Could you check a few things on this model? Use its own coordinates, in mm. Round coordinates to 2 decimals unless told otherwise and drop trailing zeros. Write each loop counter-clockwise with the first axis right and the second up, starting at its lowest first coordinate (ties: lowest second). Pieces come first, ordered by that corner, then holes. Notation, with made-up numbers: (40, -39.75) -> (88, -39.75) arc R16 cw to (88, -15.75) -> close; hole circle Ø5 at (79, -40). An arc over 180 degrees is marked (long way). Return JSON: item names as keys, results as strings.
from build123d import *

# Parameters (mm, degrees)
SKETCH_1_R      = 2
SKETCH_1_R_2    = 1.5
SKETCH_1_R_3    = 8
EXTRUDE_1_DEPTH = 2


with BuildPart() as part:
    # 草图1 → 凸台-拉伸1 (new body)
    with BuildSketch(Plane(origin=(0, 0, 0), x_dir=(1, 0, 0), z_dir=(0, 1, 0))):
        with BuildLine():
            Line((394.734384308, 186.437991397), (394.734384308, 47.57418904))
            ThreePointArc((394.734384308, 47.57418904), (392.977024848, 43.331548206), (388.734383891, 41.574189041))
            Line((388.734383891, 41.574189041), (280.734383891, 41.574189041))
            ThreePointArc((280.734383891, 41.574189041), (276.491743156, 43.331548327), (274.734383818, 47.57418904))
            Line((274.734383818, 47.57418904), (274.734383818, 186.437990955))
            ThreePointArc((274.734383818, 186.437990955), (274.374769614, 188.48397581), (273.339034443, 190.284705955))
            ThreePointArc((273.339034443, 190.284705955), (336.622100005, 321.857720451), (394.944496295, 188.011903851))
            ThreePointArc((394.944496295, 188.011903851), (394.787144273, 187.231928967), (394.734384308, 186.437991397))
        make_face()
        with Locations(Location((370.121603429, 276.574189041, 0), (0, 0, 270))):
            Circle(SKETCH_1_R, mode=Mode.SUBTRACT)
        with Locations(Location((369.73616956, 206.574189041, 0), (0, 0, 270))):
            Circle(SKETCH_1_R, mode=Mode.SUBTRACT)
        with Locations(Location((300.121603429, 206.574189041, 0), (0, 0, 270))):
            Circle(SKETCH_1_R, mode=Mode.SUBTRACT)
        with Locations(Location((313.734383891, 157.57418904, 0), (0, 0, 270))):
            Circle(SKETCH_1_R_2, mode=Mode.SUBTRACT)
        with Locations(Location((355.734383891, 157.57418904, 0), (0, 0, 270))):
            Circle(SKETCH_1_R_2, mode=Mode.SUBTRACT)
        with Locations(Location((380.234383891, 133.07418904, 0), (0, 0, 270))):
            Circle(SKETCH_1_R_2, mode=Mode.SUBTRACT)
        with Locations(Location((380.234383891, 158.07418904, 0), (0, 0, 270))):
            Circle(SKETCH_1_R_2, mode=Mode.SUBTRACT)
        with Locations(Location((364.734383891, 61.57418904, 0), (0, 0, 270))):
            Circle(SKETCH_1_R_2, mode=Mode.SUBTRACT)
        with Locations(Location((388.734383891, 61.57418904, 0), (0, 0, 270))):
            Circle(SKETCH_1_R_2, mode=Mode.SUBTRACT)
        with Locations(Location((364.734383891, 91.57418904, 0), (0, 0, 270))):
            Circle(SKETCH_1_R_2, mode=Mode.SUBTRACT)
        with Locations(Location((388.734383891, 91.57418904, 0), (0, 0, 270))):
            Circle(SKETCH_1_R_2, mode=Mode.SUBTRACT)
        with Locations(Location((304.734383891, 61.57418904, 0), (0, 0, 270))):
            Circle(SKETCH_1_R_2, mode=Mode.SUBTRACT)
        with Locations(Location((280.734383891, 61.57418904, 0), (0, 0, 270))):
            Circle(SKETCH_1_R_2, mode=Mode.SUBTRACT)
        with Locations(Location((304.734383891, 91.57418904, 0), (0, 0, 270))):
            Circle(SKETCH_1_R_2, mode=Mode.SUBTRACT)
        with Locations(Location((280.734383891, 91.57418904, 0), (0, 0, 270))):
            Circle(SKETCH_1_R_2, mode=Mode.SUBTRACT)
        with Locations(Location((334.734383891, 316.57418904, 0), (0, 0, 270))):
            Circle(SKETCH_1_R_2, mode=Mode.SUBTRACT)
        with Locations(Location((281.701375302, 294.607197629, 0), (0, 0, 270))):
            Circle(SKETCH_1_R_2, mode=Mode.SUBTRACT)
        with Locations(Location((259.734383891, 241.574189041, 0), (0, 0, 270))):
            Circle(SKETCH_1_R_2, mode=Mode.SUBTRACT)
        with Locations(Location((281.701375302, 188.541180451, 0), (0, 0, 270))):
            Circle(SKETCH_1_R_2, mode=Mode.SUBTRACT)
        with Locations(Location((387.76739248, 188.541180451, 0), (0, 0, 270))):
            Circle(SKETCH_1_R_2, mode=Mode.SUBTRACT)
        with Locations(Location((409.734383891, 241.574189041, 0), (0, 0, 270))):
            Circle(SKETCH_1_R_2, mode=Mode.SUBTRACT)
        with Locations(Location((387.76739248, 294.607197629, 0), (0, 0, 270))):
            Circle(SKETCH_1_R_2, mode=Mode.SUBTRACT)
        with Locations(Location((322.734383891, 306.575974709, 0), (0, 0, 270))):
            Circle(SKETCH_1_R_2, mode=Mode.SUBTRACT)
        with Locations(Location((346.734383891, 306.575974709, 0), (0, 0, 270))):
            Circle(SKETCH_1_R_2, mode=Mode.SUBTRACT)
        with Locations(Location((322.734383891, 276.575974709, 0), (0, 0, 270))):
            Circle(SKETCH_1_R_2, mode=Mode.SUBTRACT)
        with Locations(Location((346.734383891, 276.575974709, 0), (0, 0, 270))):
            Circle(SKETCH_1_R_2, mode=Mode.SUBTRACT)
        with Locations(Location((334.734383891, 309.57418904, 0), (0, 0, 270))):
            Circle(SKETCH_1_R_2, mode=Mode.SUBTRACT)
        with Locations(Location((341.734383891, 309.57418904, 0), (0, 0, 270))):
            Circle(SKETCH_1_R_2, mode=Mode.SUBTRACT)
        with Locations(Location((327.734383891, 309.57418904, 0), (0, 0, 270))):
            Circle(SKETCH_1_R_2, mode=Mode.SUBTRACT)
        with Locations(Location((302.217879596, 301.607197629, 0), (0, 0, 270))):
            Circle(SKETCH_1_R_2, mode=Mode.SUBTRACT)
        with Locations(Location((302.217879596, 294.607197629, 0), (0, 0, 270))):
            Circle(SKETCH_1_R_2, mode=Mode.SUBTRACT)
        with Locations(Location((309.217879596, 294.607197629, 0), (0, 0, 270))):
            Circle(SKETCH_1_R_2, mode=Mode.SUBTRACT)
        with Locations(Location((295.217879596, 294.607197629, 0), (0, 0, 270))):
            Circle(SKETCH_1_R_2, mode=Mode.SUBTRACT)
        with Locations(Location((367.250888185, 301.607197629, 0), (0, 0, 270))):
            Circle(SKETCH_1_R_2, mode=Mode.SUBTRACT)
        with Locations(Location((367.250888185, 294.607197629, 0), (0, 0, 270))):
            Circle(SKETCH_1_R_2, mode=Mode.SUBTRACT)
        with Locations(Location((360.250888185, 294.607197629, 0), (0, 0, 270))):
            Circle(SKETCH_1_R_2, mode=Mode.SUBTRACT)
        with Locations(Location((374.250888185, 294.607197629, 0), (0, 0, 270))):
            Circle(SKETCH_1_R_2, mode=Mode.SUBTRACT)
        with Locations(Location((289.234383891, 133.07418904, 0), (0, 0, 270))):
            Circle(SKETCH_1_R_2, mode=Mode.SUBTRACT)
        with Locations(Location((289.234383891, 158.07418904, 0), (0, 0, 270))):
            Circle(SKETCH_1_R_2, mode=Mode.SUBTRACT)
        with Locations(Location((304.734383891, 47.57418904, 0), (0, 0, 270))):
            Circle(SKETCH_1_R_2, mode=Mode.SUBTRACT)
        with Locations(Location((364.734383891, 47.57418904, 0), (0, 0, 270))):
            Circle(SKETCH_1_R_2, mode=Mode.SUBTRACT)
        with Locations(Location((335.121603429, 47.57418904, 0), (0, 0, 270))):
            Circle(SKETCH_1_R_2, mode=Mode.SUBTRACT)
        with Locations(Location((334.734383891, 136.57418904, 0), (0, 0, 270))):
            Circle(SKETCH_1_R_3, mode=Mode.SUBTRACT)
        with Locations(Location((300.121603429, 276.574189041, 0), (0, 0, 270))):
            Circle(SKETCH_1_R, mode=Mode.SUBTRACT)
        with Locations(Location((367.121603429, 157.57418904, 0), (0, 0, 270))):
            Circle(SKETCH_1_R_2, mode=Mode.SUBTRACT)
        with Locations(Location((367.121603429, 99.57418904, 0), (0, 0, 270))):
            Circle(SKETCH_1_R_2, mode=Mode.SUBTRACT)
        with Locations(Location((303.121603429, 157.57418904, 0), (0, 0, 270))):
            Circle(SKETCH_1_R_2, mode=Mode.SUBTRACT)
        with Locations(Location((303.121603429, 99.57418904, 0), (0, 0, 270))):
            Circle(SKETCH_1_R_2, mode=Mode.SUBTRACT)
        with BuildLine():
            Line((354.234383891, 115.57418904), (354.234383891, 89.57418904))
            ThreePointArc((354.234383891, 89.57418904), (355.734383891, 88.07418904), (357.234383891, 89.57418904))
            Line((357.234383891, 89.57418904), (357.234383891, 115.57418904))
            ThreePointArc((357.234383891, 115.57418904), (355.734383891, 117.07418904), (354.234383891, 115.57418904))
        make_face(mode=Mode.SUBTRACT)
        with BuildLine():
            Line((312.234383891, 115.57418904), (312.234383891, 89.57418904))
            ThreePointArc((312.234383891, 89.57418904), (313.734383891, 88.07418904), (315.234383891, 89.57418904))
            Line((315.234383891, 89.57418904), (315.234383891, 115.57418904))
            ThreePointArc((315.234383891, 115.57418904), (313.734383891, 117.07418904), (312.234383891, 115.57418904))
        make_face(mode=Mode.SUBTRACT)
        with BuildLine():
            Line((373.73438389, 46.07418904), (388.734383949, 46.07418904))
            ThreePointArc((388.734383949, 46.07418904), (390.234384308, 47.574188681), (388.734384668, 49.07418904))
            Line((388.734384668, 49.07418904), (373.734383891, 49.07418904))
            ThreePointArc((373.734383891, 49.07418904), (372.234383891, 47.574189041), (373.73438389, 46.07418904))
        make_face(mode=Mode.SUBTRACT)
        with BuildLine():
            Line((295.734383891, 49.07418904), (280.734383933, 49.07418904))
            ThreePointArc((280.734383933, 49.07418904), (279.234383817, 47.574189156), (280.734383701, 46.07418904))
            Line((280.734383701, 46.07418904), (295.734383891, 46.07418904))
            ThreePointArc((295.734383891, 46.07418904), (297.234383891, 47.57418904), (295.734383891, 49.07418904))
        make_face(mode=Mode.SUBTRACT)
        with BuildLine():
            Line((341.23438389, 46.07418904), (355.734383901, 46.07418904))
            ThreePointArc((355.734383901, 46.07418904), (357.234383363, 47.574189579), (355.734382825, 49.07418904))
            Line((355.734382825, 49.07418904), (341.234383891, 49.07418904))
            ThreePointArc((341.234383891, 49.07418904), (339.734383891, 47.574189041), (341.23438389, 46.07418904))
        make_face(mode=Mode.SUBTRACT)
        with BuildLine():
            Line((328.234383891, 49.07418904), (313.734383817, 49.07418904))
            ThreePointArc((313.734383817, 49.07418904), (312.234383891, 47.5741895), (313.734382898, 46.07418904))
            Line((313.734382898, 46.07418904), (328.234383891, 46.07418904))
            ThreePointArc((328.234383891, 46.07418904), (329.734383891, 47.57418904), (328.234383891, 49.07418904))
        make_face(mode=Mode.SUBTRACT)
    extrude(amount=EXTRUDE_1_DEPTH)


solid = part.part
1) I want a section at B-B, the plane x = 400.5. Please give me the cut outline in (y, z).
Return value:
{"outline": "(0, -288.19) -> (2, -288.19) -> (2, -194.95) -> (0, -194.95) -> close"}
2) Thinking about a two-plate mould opening in X: for faces 1 (the face through (393.023, 0.986, -43.378)), 2 (the face through (334.056, 0.986, -321.865)), 3 (the face through (326.925, 0.986, -138.308)), which applies, pulls with the +X half, pulls with the -X half, needs draft (parallel to the pull), parting line crosses it, or undercut?
Return value:
{"face 1": "pulls with the +X half", "face 2": "parting line crosses it", "face 3": "undercut"}
3) If I drill on probe 1 along X at (y, z) = (0.6, -108); probe 2 along Z at (x, y) = (329.5, 0.95); probe 3 along Z at (x, y) = (368, 1.1), over which ranges is the centre line in solid material (lowest first)? Write a range as [from, to].
Return value:
{"probe 1": "[274.73, 312.23], [315.23, 354.23], [357.23, 394.73]", "probe 2": "[-321.67, -142.62], [-130.52, -48.38], [-46.77, -41.57]", "probe 3": "[-314.83, -302.91], [-300.31, -295.91], [-293.31, -207.57], [-205.58, -158.79], [-156.36, -100.79], [-98.36, -41.57]"}
4) Will these pins go through, and if not, where does the flat tip stop? pin 1 Ø1.8 at (x, z) = (280.73, -61.57) entering from -Y; pin 2 Ø1 at (x, y) = (358, 0.5) entering from -Z; pin 3 Ø1 at (x, y) = (351, 1) entering from -Z.
Return value:
{"pin 1": "through", "pin 2": "z = -318.69", "pin 3": "z = -320.39"}
5) I want a section at C-C, the plane y = 0.35. Count the separate pieces of the cut face and the enclosed holes in it, and give its area (3 significant figures).
Return value:
{"separate pieces": "1", "enclosed holes": "54", "area": "34,700 mm²"}
6) I want a section at A-A, the plane z = -120. Please give me the cut outline in (x, y).
Return value:
{"outline": "(274.73, 0) -> (394.73, 0) -> (394.73, 2) -> (274.73, 2) -> close"}
